Input: part model. Units: mm. Frame: model coordinates. A direction names the side the tool comes from. Give positions to 0.01 mm unless a question says otherwise; leave off trailing zeros. Loops run counter-clockwise (first coordinate to the right, second up) from the corner with the lowest first, then second, coordinate; pieces in that order, holes last. Notation, with made-up numbers: (72.25, -5.75) - (88.25, -5.75) arc R9 ccw to (88.25, 2.25) - close; hole circle Ø4 at (39, 75). An arc over 180 degrees is marked (long way). One line per item, written item: value.
from build123d import *

# Parameters (mm, degrees)
SKETCH1_R           = 8.5
SKETCH1_R_2         = 6
BOSS_EXTRUDE1_DEPTH = 45
CUT_EXTRUDE1_REACH  = 19


with BuildPart() as part:
    # Sketch1 → Boss-Extrude1 (new body)
    with BuildSketch(Plane.XY):
        Circle(SKETCH1_R)
        Circle(SKETCH1_R_2, mode=Mode.SUBTRACT)
    extrude(amount=BOSS_EXTRUDE1_DEPTH)

    # Sketch2 → Cut-Extrude1 (cut, up to next)
    with BuildSketch(Plane(origin=(0, 8.5, 0), x_dir=(-1, 0, 0), z_dir=(0, 1, 0)), mode=Mode.PRIVATE) as cut_extrude1_sk1:
        with BuildLine():
            Line((1.5, 38.5), (1.5, 26.5))
            ThreePointArc((1.5, 26.5), (0, 25), (-1.5, 26.5))
            Line((-1.5, 26.5), (-1.5, 38.5))
            ThreePointArc((-1.5, 38.5), (0, 40), (1.5, 38.5))
        make_face()
    cut_extrude1_tool1 = extrude(cut_extrude1_sk1.sketch, amount=-CUT_EXTRUDE1_REACH, mode=Mode.PRIVATE) & part.part
    add(cut_extrude1_tool1.solids().sort_by_distance((0, 8.5, 32.5))[0], mode=Mode.SUBTRACT)


solid = part.part
Item 1: Section D-D, the plane z = 10.5. Output: boundary loops of the cut face in (x, y), and give its area (3 significant figures).
Verdict:
outline: circle Ø17 at (0, 0); hole circle Ø12 at (0, 0)
area: 114 mm^2
Item 2: Material intervals for L1, parallel to X at y = -5.25, z = 6.5; L2, parallel to Y at x = 2.25, z = 37; L3, parallel to X at y = -5, z = 7.5, sorted ascending.
Verdict:
L1: x = -6.68 to -2.9, 2.9 to 6.68
L2: y = -8.2 to -5.56, 5.56 to 8.2
L3: x = -6.87 to -3.32, 3.32 to 6.87
Item 3: Draft query along Z for faces 3 (the face through (2, 6, 45)), 4 (the face through (0, 7, 25)), 5 (the face through (2, 6, 0)), 6 (the face through (-1.5, 7, 33)). Return one class per face: pulls with the +Z half, pulls with the -Z half, needs draft (parallel to the pull), parting line crosses it, or undercut.
Verdict:
face 3: pulls with the +Z half
face 4: undercut
face 5: pulls with the -Z half
face 6: undercut
Item 4: Section C-C, the plane x = 2.5. Output: boundary loops of the cut face in (y, z), and give its area (3 significant figures).
Verdict:
outline: (-8.12, 0) - (-5.45, 0) - (-5.45, 45) - (-8.12, 45) - close; (5.45, 0) - (8.12, 0) - (8.12, 45) - (5.45, 45) - close
area: 240 mm^2
Item 5: Section B-B, the plane x = 0. Output: boundary loops of the cut face in (y, z).
Verdict:
outline: (-8.5, 0) - (-6, 0) - (-6, 45) - (-8.5, 45) - close; (6, 0) - (8.5, 0) - (8.5, 25) - (6, 25) - close; (6, 40) - (8.5, 40) - (8.5, 45) - (6, 45) - close
Item 6: Access query for faces 1 (the face through (-1.301, -5.857, 22.185)), 2 (the face through (0, 7, 40)). Directions: +Z, -Z, +X, -X, +Y, -Y. A direction counts if a zero-diameter tool reaches every point of the face in a straight line with its end or side. Return the directions, or none.
Verdict:
face 1: +Z, -Z
face 2: +Y
Item 7: Section A-A, the plane y = 0. Output: boundary loops of the cut face in (x, z).
Verdict:
outline: (-8.5, 0) - (-6, 0) - (-6, 45) - (-8.5, 45) - close; (6, 0) - (8.5, 0) - (8.5, 45) - (6, 45) - close
Item 8: Pin query (flat end, axial travel): P1, Ø2, axis at x = 1.5, z = 6, coming from the +Y side; P2, Ø5, axis at x = -5.5, z = 24, coming from the -Y side; P3, Ø1.5, axis at x = 6, z = 13.5, coming from the +Y side. Return the tip coordinate at first contact, or that it passes through.
Verdict:
P1: stops at y = 8.49
P2: stops at y = -7.95
P3: stops at y = 6.68
